```python
from build123d import *

# Parameters (mm, degrees)
SKETCH1_R           = 9
BOSS_EXTRUDE1_DEPTH = 20
BOSS_EXTRUDE4_DEPTH = 60
CUT_EXTRUDE1_START  = -45
CUT_EXTRUDE1_DEPTH  = 30
SKETCH9_R           = 12
CUT_EXTRUDE2_DEPTH  = 150.255653159


with BuildPart() as part:
    # Sketch1 → Boss-Extrude1 (new body)
    with BuildSketch(Plane(origin=(0, 0, 0), x_dir=(1, 0, 0), z_dir=(0, 1, 0))):
        with BuildLine():
            Line((-25, -72.5), (25, -72.5))
            ThreePointArc((25, -72.5), (39.142135624, -66.642135624), (45, -52.5))
            Line((45, -52.5), (45, 52.5))
            ThreePointArc((45, 52.5), (39.142135624, 66.642135624), (25, 72.5))
            Line((25, 72.5), (-25, 72.5))
            ThreePointArc((-25, 72.5), (-39.142135624, 66.642135624), (-45, 52.5))
            Line((-45, 52.5), (-45, -52.5))
            ThreePointArc((-45, -52.5), (-39.142135624, -66.642135624), (-25, -72.5))
        make_face()
        with Locations(Location((25, -52.5, 0), (0, 0, 270))):
            Circle(SKETCH1_R, mode=Mode.SUBTRACT)
        with Locations(Location((-25, -52.5, 0), (0, 0, 270))):
            Circle(SKETCH1_R, mode=Mode.SUBTRACT)
    extrude(amount=BOSS_EXTRUDE1_DEPTH)

    # Sketch4 → Boss-Extrude4 (add)
    with BuildSketch(Plane(origin=(0, 20, 0), x_dir=(1, 0, 0), z_dir=(0, 1, 0))):
        with BuildLine():
            Line((-34, -7.5), (34, -7.5))
            Line((34, -7.5), (34, 42.5))
            ThreePointArc((34, 42.5), (0, 76.5), (-34, 42.5))
            Line((-34, 42.5), (-34, -7.5))
        make_face()
    extrude(amount=BOSS_EXTRUDE4_DEPTH)

    # Sketch6 → Cut-Extrude1 (cut)
    with BuildSketch(Plane(origin=(0, 80, 0), x_dir=(1, 0, 0), z_dir=(0, 1, 0)).offset(CUT_EXTRUDE1_START)):
        with BuildLine():
            Line((-34, 12.5), (34, 12.5))
            Line((34, 12.5), (34, 42.5))
            ThreePointArc((34, 42.5), (0, 76.5), (-34, 42.5))
            Line((-34, 42.5), (-34, 12.5))
        make_face()
    extrude(amount=CUT_EXTRUDE1_DEPTH, mode=Mode.SUBTRACT)

    # Sketch7 → Revolve1 (revolve)
    with BuildSketch(Plane.XY.offset(-42.5)):
        Polygon((0, 120), (20, 120), (34, 80), (0, 80), align=None)
    revolve(axis=Axis((0, 80, -42.5), (0, 1, 0)))

    # Sketch9 → Cut-Extrude2 (cut, through all)
    with BuildSketch(Plane(origin=(0, 120, 0), x_dir=(1, 0, 0), z_dir=(0, 1, 0))):
        with Locations(Location((0, 42.5, 0), (0, 0, 180))):
            Circle(SKETCH9_R)
    extrude(amount=-CUT_EXTRUDE2_DEPTH, mode=Mode.SUBTRACT)


solid = part.part
```
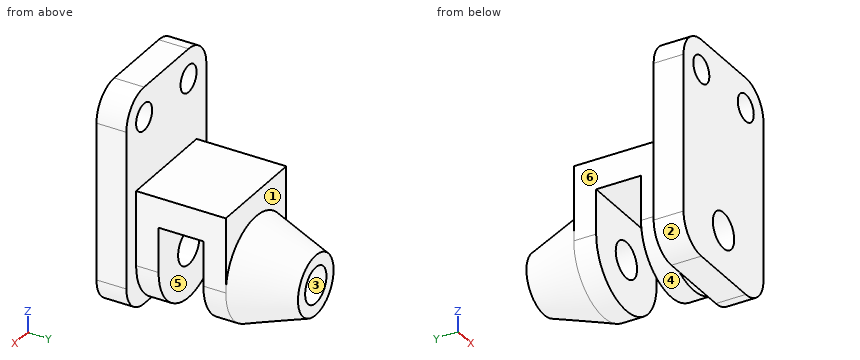
Geometry check sheet. Reference: the model listing, model coordinates, mm. Face numbers are marked on the shaded views. A direction names the side the tool comes from. Give positions to 0.01 mm unless a question says otherwise; leave off trailing zeros. Order: outer loops, then holes, each group sorted by start corner. A loop starts at its lowest first (then second) coordinate and runs counter-clockwise, first axis right, second up.
1. Thickness scan on L1, parallel to X at y = 8.25, z = 52.5; L2, parallel to Z at x = 0, y = 22; L3, parallel to Y at x = 38, z = -16. Record the ranges inside material, lowest first.
2. Access from +Z, -Z, +X, -X, +Y, -Y to the whole of each face (thin tool, end or side, straight path). Record for the marked faces 4, 5 and 6.
3. Release check for a two-part mould opening along X. For the marked faces 1, 2 and 3 record: pulls with the +X half, pulls with the -X half, needs draft (parallel to the pull), parting line crosses it, or undercut.
4. Gauge pin test, flat ends, axial feed: pin 1 Ø23.5 at (x, z) = (25, 52.5) entering from -Y; pin 2 Ø15 at (y, z) = (54.5, -16.5) entering from +X; pin 3 Ø18 at (x, y) = (8.5, 55.5) entering from +Z; pin 4 Ø22 at (x, y) = (-1.5, 7) entering from -Z. Record the tip position at first contact, or that the pin passes through.
5. Section check B-B, the plane y = 33. Enter the section's corners in (x, z).
6. Section check A-A, the plane x = 0. Enter the section's corners in (y, z).
7. Section check C-C, the plane z = -3. Enter the section's corners in (x, y), and give its area (3 significant figures).
8. Section check D-D, the plane z = 50.5. Enter the section's corners in (x, y).
Values follow:
1. L1: x = -45 to -34, -16 to 16, 34 to 45
1. L2: z = -76.5 to -54.5, -30.5 to 7.5
1. L3: y = 0 to 20
2. face 4: -Z, +Y
2. face 5: -Z, +X, -X
2. face 6: +Z, -Z, -X, +Y
3. face 1: needs draft
3. face 2: pulls with the -X half
3. face 3: undercut
4. pin 1: stops at y = 0
4. pin 2: stops at x = 34
4. pin 3: stops at z = 7.5
4. pin 4: stops at z = -72.5
5. outline: (-34, -42.5) arc R34 ccw to (34, -42.5) - (34, 7.5) - (-34, 7.5) - close; hole circle Ø24 at (0, -42.5)
6. outline: (0, -72.5) - (20, -72.5) - (20, -76.5) - (35, -76.5) - (35, -54.5) - (0, -54.5) - close; (0, -30.5) - (35, -30.5) - (35, -12.5) - (65, -12.5) - (65, -30.5) - (120, -30.5) - (120, -22.5) - (80, -8.5) - (80, 7.5) - (20, 7.5) - (20, 72.5) - (0, 72.5) - close; (65, -76.5) - (80, -76.5) - (120, -62.5) - (120, -54.5) - (65, -54.5) - close
7. outline: (-45, 0) - (45, 0) - (45, 20) - (34, 20) - (34, 80) - (-34, 80) - (-34, 20) - (-45, 20) - close
7. area: 5,880 mm2
8. outline: (-45, 0) - (-33.77, 0) - (-33.77, 20) - (-45, 20) - close; (-16.23, 0) - (16.23, 0) - (16.23, 20) - (-16.23, 20) - close; (33.77, 0) - (45, 0) - (45, 20) - (33.77, 20) - close
